Work out the finished part from the listing and answer in its coordinate system (mm). A direction names the side the tool comes from. Round coordinates to 2 decimals unless told otherwise and drop trailing zeros. Order: outer loops, then holes, each group sorted by start corner. A loop starts at its lowest first (then second) coordinate and runs counter-clockwise, first axis right, second up. Notation, with made-up numbers: (7.5, 18) -> (26.5, 18) arc R26 cw to (26.5, 55) -> close; hole circle Ø1 at (-11.5, -30). An arc over 180 degrees is marked (long way). Use one line per item in the form item = value.
```python
from build123d import *

# Parameters (mm, degrees)
CROQUIS1_W              = 29
CROQUIS1_H              = 17
SALIENTE_EXTRUIR1_DEPTH = 43
CROQUIS2_R              = 10
SALIENTE_EXTRUIR2_DEPTH = 29
CROQUIS3_R              = 2.1
CORTAR_EXTRUIR1_DEPTH   = 29
SALIENTE_EXTRUIR3_DEPTH = 29


with BuildPart() as part:
    # Croquis1 → Saliente-Extruir1 (new body)
    with BuildSketch(Plane(origin=(0, 0, 0), x_dir=(1, 0, 0), z_dir=(0, 1, 0))):
        with Locations((14.5, -8.5)):
            Rectangle(CROQUIS1_W, CROQUIS1_H)
    extrude(amount=SALIENTE_EXTRUIR1_DEPTH)



with BuildPart() as body_2:
    # Croquis2 → Saliente-Extruir2 (new body)
    with BuildSketch(Plane(origin=(29, 0, 0), x_dir=(0, 0, -1), z_dir=(1, 0, 0))):
        with Locations((-34, 39)):
            Circle(CROQUIS2_R)
    extrude(amount=-SALIENTE_EXTRUIR2_DEPTH)

    # Croquis3 → Cortar-Extruir1 (cut)
    with BuildSketch(Plane(origin=(29, 0, 0), x_dir=(0, 0, -1), z_dir=(1, 0, 0))):
        with Locations((-34, 39)):
            Circle(CROQUIS3_R)
    extrude(amount=-CORTAR_EXTRUIR1_DEPTH, mode=Mode.SUBTRACT)


with BuildPart() as part_1:
    add(part.part)

    add(body_2.part)  # Saliente-Extruir3 merges body 2
    # Croquis4 → Saliente-Extruir3 (add)
    with BuildSketch(Plane(origin=(29, 0, 0), x_dir=(0, 0, -1), z_dir=(1, 0, 0))):
        with BuildLine():
            Line((-34, 29), (-17, 29))
            Line((-17, 29), (-17, 43))
            ThreePointArc((-17, 43), (-21.814511478, 43.643262372), (-26.334473676, 45.421814866))
            ThreePointArc((-26.334473676, 45.421814866), (-24.938594241, 34.770233379), (-34, 29))
        make_face()
    extrude(amount=-SALIENTE_EXTRUIR3_DEPTH)


solid = part_1.part
```
Item 1: Flat-ended cylindrical pins translate along their axes: P1, Ø8, axis at x = 10.5, z = 17.5, coming from the +Y side; P2, Ø10, axis at x = 15, z = 37.5, coming from the -Y side; P3, Ø1, axis at y = 27.5, z = 36, coming from the -X side; P4, Ø14.5, axis at x = 12, y = 16.5, coming from the +Z side. Find the tip coordinate at first contact, or state that the pin passes through.
Findings:
P1 = 43.56
P2 = 29
P3 = through
P4 = 17
Item 2: The part is cut by section B-B, the plane x = 8.5. Give the vertices of the cut face in (y, z).
Findings:
outline = (0, 0) -> (43, 0) -> (43, 17) arc R20.12 cw to (45.42, 26.33) arc R10 ccw (long way) to (29, 34) -> (29, 17) -> (0, 17) -> close; hole circle Ø4.2 at (39, 34)
Item 3: Determine the mould class of faces 4 (the cylindrical face through (14.703, 37.722, 35.666)), 5 (the cylindrical face through (14.703, 43.626, 21.748)), 6 (the flat face through (14, 0, 8)) for opening direction Z: released by +Z, released by -Z, zero draft, split by the parting line, or undercut.
Findings:
face_4 = undercut
face_5 = released by -Z
face_6 = zero draft
Item 4: The part is cut by section D-D, the plane y = 13.5. Give the vertices of the cut face in (x, z).
Findings:
outline = (0, 0) -> (29, 0) -> (29, 17) -> (0, 17) -> close
Item 5: The part is cut by section A-A, the plane y = 39. Give the vertices of the cut face in (x, z).
Findings:
outline = (0, 0) -> (29, 0) -> (29, 31.9) -> (0, 31.9) -> close; (0, 36.1) -> (29, 36.1) -> (29, 44) -> (0, 44) -> close
Item 6: Consider line 1 along Y through (x, z) = (6.5, 34); line 2 along Y through (x, z) = (2, 8); line 3 along Z through (x, y) = (13.5, 25.5). Determine where each line is inside the solid, lowest interval first.
Findings:
line_1 = 29 to 36.9, 41.1 to 49
line_2 = 0 to 43
line_3 = 0 to 17
Item 7: The part is cut by section C-C, the plane z = 33. Give the vertices of the cut face in (x, y), and give its area (3 significant figures).
Findings:
outline = (0, 29) -> (29, 29) -> (29, 37.15) -> (0, 37.15) -> close; (0, 40.85) -> (29, 40.85) -> (29, 48.95) -> (0, 48.95) -> close
area = 471 mm^2
Item 8: For faces 1 (the flat face through (14, 21, 0)), 2 (the flat face through (14, 14, 17)), 3 (the flat face through (14, 43, 8)), determine the directions among +Z, -Z, +X, -X, +Y, -Y from which every point of the face is accessible in a straight line to the end or side of a thin tool.
Findings:
face_1 = -Z, +X, -X, +Y, -Y
face_2 = +Z, +X, -X, -Y
face_3 = -Z, +X, -X, +Y
